Read the model definition and answer for the solid it produces. Units are mm, in the model's axes. Face numbers are marked on the shaded views. Coordinates: 2 decimals unless noted, no trailing zeros. Loops run counter-clockwise (first coordinate to the right, second up) from the corner with the lowest first, then second, coordinate; pieces in that order, holes last. Notation, with made-up numbers: (72.25, -16) - (107.25, -16) arc R24 cw to (107.25, 4) - close; hole circle Ø6 at (47, 59). An arc over 180 degrees is marked (long way). Use one line per item in the form item = value.
from build123d import *

# Parameters (mm, degrees)
PAD_DEPTH    = 10
SKETCH001_R  = 2.5
POCKET_DEPTH = 3


with BuildPart() as part:
    # Sketch → Pad (new body)
    with BuildSketch(Plane.XZ):
        with BuildLine():
            ThreePointArc((30, 3), (0, 30.149627), (-30, 3))
            Line((-30, 3), (-40, 3))
            Line((-40, 3), (-40, 0))
            Line((-40, 0), (-27, 0))
            Line((-27, 3), (-27, 0))
            ThreePointArc((27, 3), (0, 27.166155), (-27, 3))
            Line((27, 3), (27, 0))
            Line((27, 0), (40, 0))
            Line((40, 0), (40, 3))
            Line((40, 3), (30, 3))
        make_face()
    extrude(amount=PAD_DEPTH)

    # Sketch001 (on Face6 of Pad) → Pocket (cut)
    with BuildSketch(Plane(origin=(0, 0, 3), x_dir=(-1, 0, 0), z_dir=(0, 0, 1))):
        with Locations((-35, 5)):
            Circle(SKETCH001_R)
        with Locations((35, 5)):
            Circle(SKETCH001_R)
    extrude(amount=-POCKET_DEPTH, mode=Mode.SUBTRACT)


solid = part.part
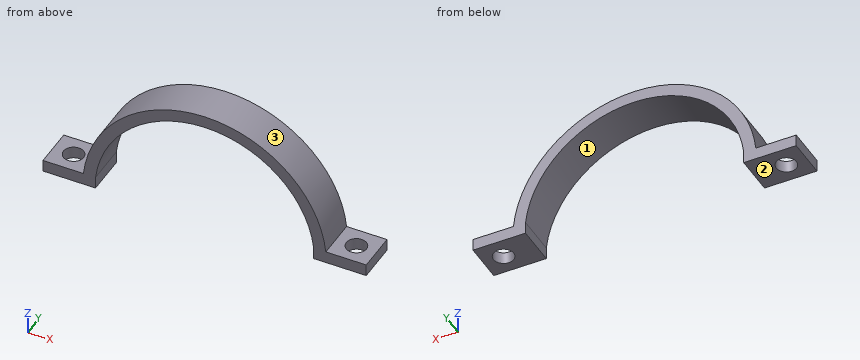
Item 1: The part is cut by section D-D on y = -0.75. Give the vertices of the cut face in (x, z), plus the area to 3 significant figures.
Results below:
outline = (-40, 0) - (-27, 0) - (-27, 3) arc R27.17 cw to (27, 3) - (27, 0) - (40, 0) - (40, 3) - (30, 3) arc R30.15 ccw to (-30, 3) - (-40, 3) - close
area = 329 mm²
Item 2: The part is cut by section B-B on x = -35. Give the vertices of the cut face in (y, z), plus the area to 3 significant figures.
Results below:
outline = (-10, 0) - (-7.5, 0) - (-7.5, 3) - (-10, 3) - close; (-2.5, 0) - (0, 0) - (0, 3) - (-2.5, 3) - close
area = 15.0 mm²
Item 3: The part is cut by section C-C on z = 13. Give the vertices of the cut face in (x, y), plus the area to 3 significant figures.
Results below:
outline = (-27.2, -10) - (-23.85, -10) - (-23.85, 0) - (-27.2, 0) - close; (23.85, -10) - (27.2, -10) - (27.2, 0) - (23.85, 0) - close
area = 67.0 mm²
Item 4: Find the intervals of material crossed by L1, parallel to X at y = -5, z = 1.35; L2, parallel to Y at x = -35, z = 2; L3, parallel to Z at x = 35.5, y = -1.75, in increasing order.
Results below:
L1 = -40 to -37.5, -32.5 to -27, 27 to 32.5, 37.5 to 40
L2 = -10 to -7.5, -2.5 to 0
L3 = 0 to 3
Item 5: Each of these flat-tipped pins is pushed along its axis until it touches: P1, Ø5, axis at y = -4, z = 6.5, coming from the -X side; P2, Ø3, axis at x = 37, y = -3.5, coming from the +Z side; P3, Ø10, axis at x = 31, z = 18, coming from the +Y side; P4, Ø2, axis at x = 7.5, y = -7.5, coming from the +Z side. Where does it stop, or does it pass through?
Results below:
P1 = -29.88
P2 = 3
P3 = through
P4 = 29.44
Item 6: The part is cut by section A-A on y = -5. Give the vertices of the cut face in (x, z).
Results below:
outline = (-40, 0) - (-37.5, 0) - (-37.5, 3) - (-40, 3) - close; (-32.5, 0) - (-27, 0) - (-27, 3) arc R27.17 cw to (27, 3) - (27, 0) - (32.5, 0) - (32.5, 3) - (30, 3) arc R30.15 ccw to (-30, 3) - (-32.5, 3) - close; (37.5, 0) - (40, 0) - (40, 3) - (37.5, 3) - close
Item 7: For a pull along X with two mould halves and no side action, classify the marked faces 1, 2 and 3 as +X half, -X half, draft (parallel to the pull), parting line (faces both ways), or undercut.
Results below:
face_1 = undercut
face_2 = draft
face_3 = parting line
